The model under review builds one solid part; all positions refer to its coordinate system, in mm. Face numbers are marked on the shaded views. A direction names the side the tool comes from. Round coordinates to 2 decimals unless told otherwise and drop trailing zeros. Loops run counter-clockwise (first coordinate to the right, second up) from the corner with the lowest first, then second, coordinate; pieces in that order, holes last. Notation, with made-up numbers: M 78,-5 L 99,-5 A8 ccw 99,7 Z; hole C 28,-23 d2. An arc over 180 degrees is marked long. Use a Markdown table: item, result. Add a question column.
```python
from build123d import *

# Parameters (mm, degrees)
FILLET1_R            = 0.2
FILLET1_OF_MIRROR1_R = 0.2


with BuildPart() as part:
    # Sketch1 → Revolve1 (revolve)
    with BuildSketch(Plane(origin=(0, 0, 0), x_dir=(0, 0, -1), z_dir=(1, 0, 0))):
        Polygon((-6, 0), (-6, 2), (-5.3, 2), (-5.3, 1.8), (-3.9, 1.8), (-3.9, 2), (-3, 2), (-3, 0), align=None)
    revolve1 = revolve(axis=Axis((0, 15.203883495, 0), (0, -1, 0)))

    # Fillet1
    fillet1_edges = [part.edges().sort_by_distance(p)[0] for p in [
        (0, 2, -3),
        (0, 2, -6),
    ]]
    fillet(fillet1_edges, radius=FILLET1_R)

    # Mirror1: Revolve1 across plane
    add(revolve1.mirror(Plane.ZX))

    # Fillet1 of Mirror1
    fillet1_of_mirror1_edges = [part.edges().sort_by_distance(p)[0] for p in [
        (0, -2, -3),
        (0, -2, -6),
    ]]
    fillet(fillet1_of_mirror1_edges, radius=FILLET1_OF_MIRROR1_R)


solid = part.part
```
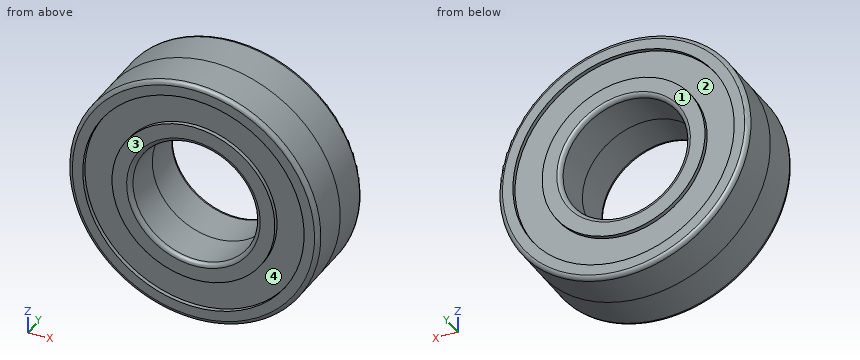
(1) To check wall thickness, follow probe 1 along Z at (x, y) = (0, -1.35); probe 2 along X at (y, z) = (1.9, 0). State the ranges of each line that lie inside material, in increasing order.
(2) Draft analysis for pull direction X (two halves, no side actions). For the marked faces 3 and 4, state which applies: released by +X, released by -X, zero draft, split by the parting line, or undercut.
(3) For the marked faces 1 and 2, list the 3-axis set-ups (+Z, -Z, +X, -X, +Y, -Y) from which the entire face can be reached by the end or side of a thin tool; tool diameter is ignored.
(4) Consider section C-C, the plane y = -0.4. Give the boundary of the cut face in (x, z), then the cut area to 3 significant figures.
(5) Insertion check: pin 1 Ø2 at (y, z) = (-0.5, -2.5) entering from +X; pin 2 Ø1 at (y, z) = (-1, -3) entering from +X. Each pin has a flat end and moves straight along its axis. Give the tip position at first contact, or say it passes through.
Found:
| question | item | result |
|---|---|---|
| 1 | probe 1 | z = -6 to -3, 3 to 6 |
| 1 | probe 2 | x = -5.97 to -5.3, -3.9 to -3.03, 3.03 to 3.9, 5.3 to 5.97 |
| 2 | face 3 | zero draft |
| 2 | face 4 | undercut |
| 3 | face 1 | +Z, -Z, +X, -X, +Y |
| 3 | face 2 | +Y |
| 4 | outline | C 0,0 d12; hole C 0,0 d6 |
| 4 | area | 84.8 mm^2 |
| 5 | pin 1 | stops at x = 5.81 |
| 5 | pin 2 | stops at x = 5.45 |
